```python
from build123d import *

# Parameters (mm, degrees)
BASE_FLANGE2_DEPTH           = 1.5
EDGE_FLANGE1_STRIP_W         = 10
EDGE_FLANGE1_STRIP_H         = 1.5
EDGE_FLANGE1_STRIP_CUT_DEPTH = 580
EDGE_FLANGE1_DEPTH           = 580
CUT_EXTRUDE1_DEPTH           = 295.957624075


# Sheet-metal steps are written as plain solids
with BuildPart() as part:
    # Sketch1 → Base-Flange2 (new body)
    with BuildSketch(Plane.XY):
        Polygon((-290, 10), (290, 10), (290, -5), (50, -50), (-50, -50), (-290, -5), align=None)
    extrude(amount=-BASE_FLANGE2_DEPTH)

    # Edge-Flange1 strip (across the edge) → Edge-Flange1 strip cut (cut)
    with BuildSketch(Plane(origin=(-290, 10, -1.5), x_dir=(0, -1, 0), z_dir=(1, 0, 0))):
        with Locations((-1.5, -0.75)):
            Rectangle(EDGE_FLANGE1_STRIP_W, EDGE_FLANGE1_STRIP_H)
    extrude(amount=EDGE_FLANGE1_STRIP_CUT_DEPTH, mode=Mode.SUBTRACT)

    # Edge-Flange1 section (across the edge) → Edge-Flange1 (add)
    with BuildSketch(Plane(origin=(-290, 10, -1.5), x_dir=(0, -1, 0), z_dir=(1, 0, 0))):
        with BuildLine():
            Line((0, 2), (0, 18.5))
            Line((0, 18.5), (1.5, 18.5))
            Line((1.5, 18.5), (1.5, 2))
            ThreePointArc((1.5, 2), (2.085786438, 0.585786438), (3.5, 0))
            Line((3.5, 0), (3.5, -1.5))
            ThreePointArc((3.5, -1.5), (1.025126266, -0.474873734), (0, 2))
        make_face()
    extrude(amount=EDGE_FLANGE1_DEPTH)

    # Sketch13 → Cut-Extrude1 (cut, through all)
    with BuildSketch(Plane.XY):
        with BuildLine():
            Line((-13.5, -3.5), (-13.5, 21.0126417))
            Line((-13.5, 21.0126417), (13.5, 21.0126417))
            Line((13.5, 21.0126417), (13.5, -3.5))
            ThreePointArc((13.5, -3.5), (0, -17), (-13.5, -3.5))
        make_face()
    extrude(amount=-CUT_EXTRUDE1_DEPTH, mode=Mode.SUBTRACT)


solid = part.part
```
Verification items for the finished model (mm, model axes). A direction names the side the tool comes from. Coordinates: 2 decimals unless noted, no trailing zeros. Loops run counter-clockwise (first coordinate to the right, second up) from the corner with the lowest first, then second, coordinate; pieces in that order, holes last. Notation, with made-up numbers: (80, 50) -> (86, 50) arc R14 cw to (86, 65) -> close; hole circle Ø1 at (-40, -25.5). An arc over 180 degrees is marked (long way). Put each result on its own line as item: value.
1. Section check C-C, the plane y = -38. Record the boundary of the cut face in (x, z).
Result set:
outline: (-114, -1.5) -> (114, -1.5) -> (114, 0) -> (-114, 0) -> close
2. Thickness scan on line 1 (Z direction, x = 24.5, y = -13.5); line 2 (Y direction, x = -132.5, z = -18.25); line 3 (Y direction, x = 250.5, z = -1.25). Record the ranges inside material, lowest first.
Result set:
line 1: z = -1.5 to 0
line 2: y = 8.5 to 10
line 3: y = -12.41 to 9.18
3. Section check D-D, the plane x = 0. Record the boundary of the cut face in (y, z).
Result set:
outline: (-50, -1.5) -> (-17, -1.5) -> (-17, 0) -> (-50, 0) -> close
4. Mould release check, pull along X, two halves, no side actions. Record for faces 1 (the face through (290, 9, -6)), 2 (the face through (0, -17, -1)), 3 (the face through (-13.5, 9, -7)), 4 (the face through (-154, 10, -12)): pulls with the +X half, pulls with the -X half, needs draft (parallel to the pull), parting line crosses it, or undercut.
Result set:
face 1: pulls with the +X half
face 2: undercut
face 3: undercut
face 4: needs draft
5. Tool access check on faces 5 (the face through (13.5, 9, -7)), 6 (the face through (-168.32, -27.815, -0.74)), 7 (the face through (-154, 8.5, -12)). Record the directions out of +Z, -Z, +X, -X, +Y, -Y that give a thin tool (end or side, any length) a straight path to the whole face; none if there is none.
Result set:
face 5: +Z, -Z, +Y
face 6: +Z, -Z, -X, -Y
face 7: -Z, +X, -X, -Y
6. Section check B-B, the plane x = -165. Record the boundary of the cut face in (y, z).
Result set:
outline: (-28.44, -1.5) -> (6.5, -1.5) arc R2 cw to (8.5, -3.5) -> (8.5, -20) -> (10, -20) -> (10, -3.5) arc R3.5 ccw to (6.5, 0) -> (-28.44, 0) -> close
7. Section check A-A, the plane z = -8.5. Record the boundary of the cut face in (x, y), then the cut area to 4 significant figures.
Result set:
outline: (-290, 8.5) -> (-13.5, 8.5) -> (-13.5, 10) -> (-290, 10) -> close; (13.5, 8.5) -> (290, 8.5) -> (290, 10) -> (13.5, 10) -> close
area: 829.5 mm^2
8. Gauge pin test, flat ends, axial feed: P1, Ø6, axis at x = -172.5, z = -8, coming from the -Y side; P2, Ø5, axis at x = 192.5, y = -25.5, coming from the -Z side; P3, Ø1.5, axis at x = 182, z = -2.5, coming from the +Y side. Record the tip position at first contact, or that the pin passes through.
Result set:
P1: stops at y = 8.5
P2: stops at z = -1.5
P3: stops at y = 9.99
